Can you work these out from the model? Positions are in its coordinate system, mm. Round coordinates to 2 decimals unless told otherwise and drop trailing zeros. Order: outer loops, then holes, each group sorted by start corner. A loop starts at its lowest first (then second) coordinate and runs counter-clockwise, first axis right, second up. Notation, with made-up numbers: M 49.5,33.5 L 105.5,33.5 A17 ccw 105.5,50.5 Z; hole C 65.5,-37 d11. An arc over 180 degrees is marked long. Answer as CSV lines item,"result". Start each with the question number.
from build123d import *

# Parameters (mm, degrees)
SKETCH1_R           = 50.8
BOSS_EXTRUDE1_DEPTH = 38.1
BOSS_EXTRUDE1_DRAFT = -7.5
SKETCH2_R           = 14.2875
CUT_EXTRUDE1_DEPTH  = 38.1
SKETCH3_R           = 3.175
CUT_EXTRUDE2_DEPTH  = 38.1


with BuildPart() as part:
    # Sketch1 → Boss-Extrude1 (with draft: the straight prism first)
    with BuildSketch(Plane.XY):
        Circle(SKETCH1_R)
    extrude(amount=BOSS_EXTRUDE1_DEPTH)
    # Boss-Extrude1: the draft: its side faces are tilted about the plane it starts from
    boss_extrude1_sides = [part.faces().sort_by_distance(p)[0] for p in [
        (-50.8, 0, 19.05),
    ]]
    draft(boss_extrude1_sides, Plane.XY, BOSS_EXTRUDE1_DRAFT)

    # Sketch2 → Cut-Extrude1 (cut)
    with BuildSketch(Plane(origin=(0, 0, 0), x_dir=(-1, 0, 0), z_dir=(0, 0, -1))):
        Circle(SKETCH2_R)
    extrude(amount=-CUT_EXTRUDE1_DEPTH, mode=Mode.SUBTRACT)

    # Sketch3 → Cut-Extrude2 (cut)
    with BuildSketch(Plane(origin=(0, 0, 0), x_dir=(-1, 0, 0), z_dir=(0, 0, -1))):
        with Locations((34.925, 0)):
            Circle(SKETCH3_R)
        with Locations((17.4625, -30.245937227)):
            Circle(SKETCH3_R)
        with Locations((-17.4625, -30.245937227)):
            Circle(SKETCH3_R)
        with Locations((-34.925, 0)):
            Circle(SKETCH3_R)
        with Locations((-17.4625, 30.245937227)):
            Circle(SKETCH3_R)
        with Locations((17.4625, 30.245937227)):
            Circle(SKETCH3_R)
    extrude(amount=-CUT_EXTRUDE2_DEPTH, mode=Mode.SUBTRACT)


solid = part.part
(1) I want a section at B-B on y = 0. Write out the boundary of the cut face in (x, z).
(2) I'm going to push flat-ended pins straight in: P1, Ø4, axis at x = 31, z = 30, coming from the -Y side; P2, Ø10, axis at y = 35, z = 14.5, coming from the +X side; P3, Ø1.5, axis at y = -17, z = 8, coming from the +X side. Where does each tip first touch, or does it pass through?
(3) If I drill on line 1 along Y through (x, z) = (17, 19); line 2 along X through (y, z) = (9, 34.5); line 3 along X through (y, z) = (-5.5, 7), over which ranges is the centre line in solid material (lowest first)?
(4) If we mould it in two halves opening along Y, with no side actions, what happens to faces 1 (the flat face through (11, -11, 0)), 2 (the cylindrical face through (-20.395, 29.03, 18.783)), 3 (the conical face through (49.75, 15.67, 10.32))? For each: +Y half, -Y half, draft (parallel to the pull), parting line (faces both ways), or undercut.
(5) I want a section at C-C on z = 17.5. Count the separate pieces of the cut face and the enclosed holes in it, and give its area (3 significant figures).
(6) I want a section at A-A on x = 0. Write out the boundary of the cut face in (y, z).
From the geometry:
1,outline,"M -55.82,38.1 L -50.8,0 L -38.1,0 L -38.1,38.1 Z; M -31.75,0 L -14.29,0 L -14.29,38.1 L -31.75,38.1 Z; M 14.29,0 L 31.75,0 L 31.75,38.1 L 14.29,38.1 Z; M 38.1,0 L 50.8,0 L 55.82,38.1 L 38.1,38.1 Z"
2,P1,"y = -46.48"
2,P2,"x = 43.43"
2,P3,"x = 49.26"
3,line 1,"-50.52 to -33.39, -27.1 to 27.1, 33.39 to 50.52"
3,line 2,"-54.61 to -11.1, 11.1 to 54.61"
3,line 3,"-51.43 to -13.19, 13.19 to 51.43"
4,face 1,"draft"
4,face 2,"undercut"
4,face 3,"parting line"
5,separate pieces,"1"
5,enclosed holes,"7"
5,area,"8,030 mm²"
6,outline,"M -55.82,38.1 L -50.8,0 L -14.29,0 L -14.29,38.1 Z; M 14.29,0 L 50.8,0 L 55.82,38.1 L 14.29,38.1 Z"
